Here's the drawing with two shaded views (mm, measured from the low corner). I have some questions. Round coordinates to 2 decimals unless told otherwise and drop trailing zeros. Order: outer loops, then holes, each group sorted by start corner. A loop starts at its lowest first (then second) coordinate and runs counter-clockwise, first axis right, second up. Notation, with made-up numbers: (47, 84.5) - (88, 84.5) arc R7 cw to (88, 90.5) - close; hole circle Ø4 at (77.5, 31). An arc over 180 degrees is marked (long way). One line per item, written item: value.
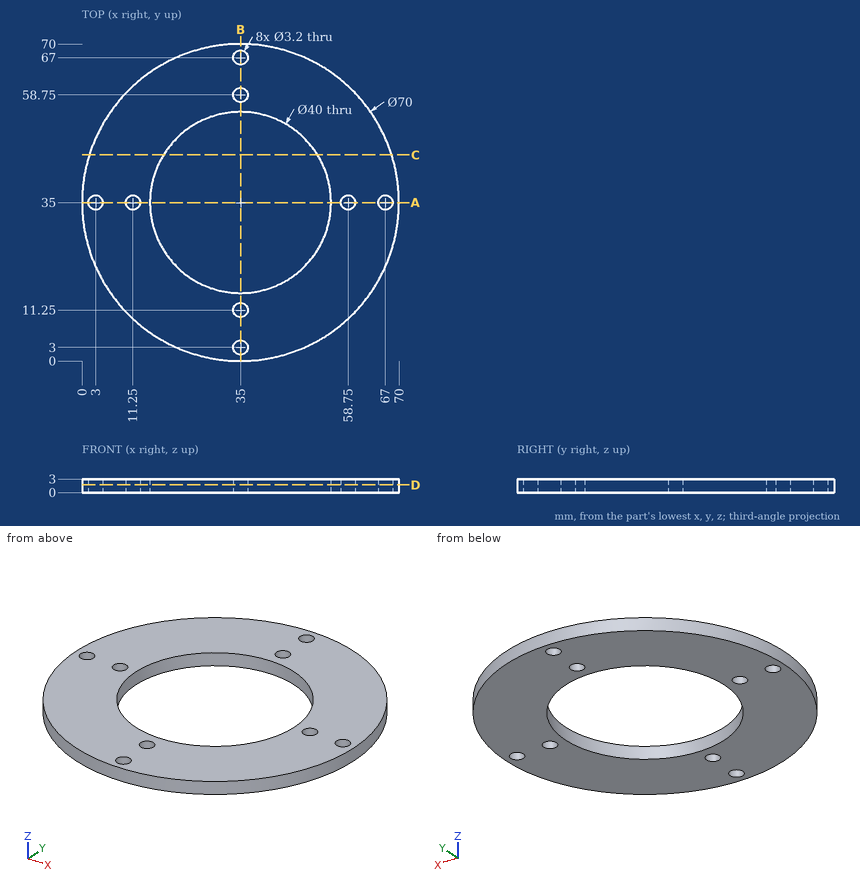
Q1. If we section it at D-D, the plane z = 1.7: Give the number of separate pieces and of enclosed holes in the cut face, then the cut area to 3 significant figures.
Results list:
separate pieces: 1
enclosed holes: 9
area: 2,530 mm²
Q2. If we section it at A-A, the plane y = 35: Please give me the cut outline in (x, z), then the cut area to 3 significant figures.
Results list:
outline: (0, 0) - (1.4, 0) - (1.4, 3) - (0, 3) - close; (4.6, 0) - (9.65, 0) - (9.65, 3) - (4.6, 3) - close; (12.85, 0) - (15, 0) - (15, 3) - (12.85, 3) - close; (55, 0) - (57.15, 0) - (57.15, 3) - (55, 3) - close; (60.35, 0) - (65.4, 0) - (65.4, 3) - (60.35, 3) - close; (68.6, 0) - (70, 0) - (70, 3) - (68.6, 3) - close
area: 51.6 mm²
Q3. If I drill on line 1 along Y through (x, z) = (35, 1.2); line 2 along X through (y, z) = (58.75, 2.3); line 3 along Y through (x, z) = (29.5, 1.8), over which ranges is the centre line in solid material (lowest first)?
Results list:
line 1: 0 to 1.4, 4.6 to 9.65, 12.85 to 15, 55 to 57.15, 60.35 to 65.4, 68.6 to 70
line 2: 9.29 to 33.4, 36.6 to 60.71
line 3: 0.43 to 15.77, 54.23 to 69.57
Q4. Will these pins go through, and if not, where does the flat tip stop? pin 1 (1 mm diameter, centred on x = 57, z = 2, fed in from +Y); pin 2 (24 mm diameter, centred on x = 35, y = 35, fed in from +Z).
Results list:
pin 1: y = 62.62
pin 2: through
Q5. If we section it at C-C, the plane y = 45.5: Please give me the cut outline in (x, z).
Results list:
outline: (1.61, 0) - (17.98, 0) - (17.98, 3) - (1.61, 3) - close; (52.02, 0) - (68.39, 0) - (68.39, 3) - (52.02, 3) - close
